Read the model definition and answer for the solid it produces. Units are mm, in the model's axes. Face numbers are marked on the shaded views. A direction names the side the tool comes from. Give positions to 0.01 mm unless a question says otherwise; leave off trailing zeros. Loops run counter-clockwise (first coordinate to the right, second up) from the corner with the lowest first, then second, coordinate; pieces in that order, holes last. Notation, with made-up numbers: (25.25, 41) -> (48.25, 41) arc R30 cw to (48.25, 68) -> close; hole circle Ø3 at (-39.5, 27). An arc over 180 degrees is marked (long way). Write each question's results on one line, items separated by ' | '. Start each with the question number.
Item 1: Section A-A on x = 74 is taken. Write down the section's boundary in (y, z), and give its area (3 significant figures).
Item 2: Each of these flat-tipped pins is pushed along its axis until it touches: P1, Ø14, axis at x = 20, y = 1, coming from the -Z side; P2, Ø1.3, axis at x = 16.5, y = 17.5, coming from the -Z side; P3, Ø10, axis at x = 48, y = 4.5, coming from the -Z side; P4, Ø12, axis at y = 2.5, z = -10, coming from the +X side. Where does it stop, or does it pass through?
Item 3: Which of the six approach directions +Z, -Z, +X, -X, +Y, -Y give full straight-line access (tool end or side, diameter ignored) to the marked faces 1, 2 and 3?
Item 4: Find the intervals of material crossed by line 1 (Y direction, x = 20.5, z = -11); line 2 (Z direction, x = 29.5, y = 4.25); line 3 (Z direction, x = 51.5, y = 13.25), in increasing order.
Item 5: Section B-B on z = -11 is taken. Write down the section's boundary in (x, y).
Item 6: Section C-C on y = 3.5 is taken. Write down the section's boundary in (x, z).
```python
from build123d import *

# Parameters (mm, degrees)
F0_W     = 80
F0_H     = 20
F1_DEPTH = 2
F2_W     = 98
F2_H     = 3
F3_DEPTH = 24
F4_R     = 2.5


with BuildPart() as f1:
    # F0 (on Top) → F1 (new body)
    with BuildSketch(Plane.XY):
        with Locations((40, 10)):
            Rectangle(F0_W, F0_H)
        Polygon((-18, -5), (0, 0), (0, 20), (-18, 20), align=None)
    extrude(amount=F1_DEPTH)

    # F2 (on face) → F3 (join)
    with BuildSketch(Plane(origin=(0, 0, 0), x_dir=(1, 0, 0), z_dir=(0, 0, -1))):
        with Locations((31, -11.5)):
            Rectangle(F2_W, F2_H)
    extrude(amount=F3_DEPTH)

    # F4
    f4_edges = [f1.edges().sort_by_distance(p)[0] for p in [
        (31, 10, 0),
        (31, 13, 0),
    ]]
    fillet(f4_edges, radius=F4_R)


solid = f1.part
```
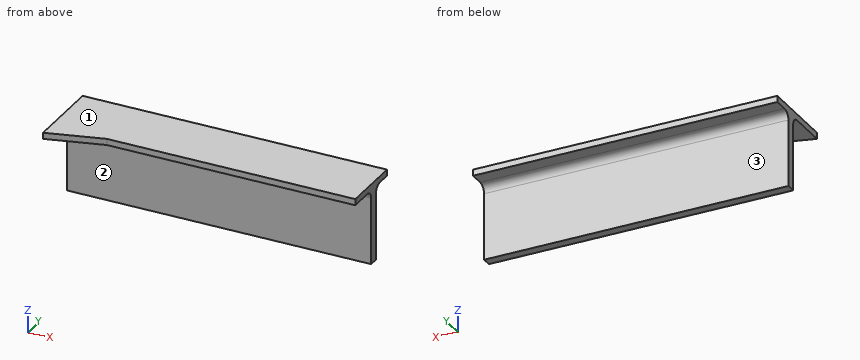
Findings:
1) outline: (0, 0) -> (7.5, 0) arc R2.5 cw to (10, -2.5) -> (10, -24) -> (13, -24) -> (13, -2.5) arc R2.5 cw to (15.5, 0) -> (20, 0) -> (20, 2) -> (0, 2) -> close | area: 115 mm2
2) P1: z = -0.05 | P2: z = 0 | P3: z = -1 | P4: through
3) face 1: +Z, +X, -X, +Y, -Y | face 2: -Z, +X, -X, -Y | face 3: -Z, +X, -X, +Y
4) line 1: 10 to 13 | line 2: 0 to 2 | line 3: -1.41 to 2
5) outline: (-18, 10) -> (80, 10) -> (80, 13) -> (-18, 13) -> close
6) outline: (-18, 0) -> (80, 0) -> (80, 2) -> (-18, 2) -> close
